```python
from build123d import *

# Parameters (mm, degrees)
BOSS_EXTRUDE1_DEPTH = 180
SKETCH3_R           = 3
SKETCH3_R_2         = 3.5
CUT_EXTRUDE1_DEPTH  = 95
SKETCH4_R           = 6
CUT_EXTRUDE2_DEPTH  = 95


with BuildPart() as part:
    # Sketch1 → Boss-Extrude1 (new body)
    with BuildSketch(Plane(origin=(0, 0, 0), x_dir=(1, 0, 0), z_dir=(0, 1, 0))):
        with BuildLine():
            Line((-20.4, 25.4), (20.4, 25.4))
            ThreePointArc((20.4, 25.4), (23.935533906, 23.935533906), (25.4, 20.4))
            Line((25.4, 20.4), (25.4, -20.4))
            ThreePointArc((25.4, -20.4), (23.935533906, -23.935533906), (20.4, -25.4))
            Line((20.4, -25.4), (-20.4, -25.4))
            ThreePointArc((-20.4, -25.4), (-23.935533906, -23.935533906), (-25.4, -20.4))
            Line((-25.4, -20.4), (-25.4, 20.4))
            ThreePointArc((-25.4, 20.4), (-23.935533906, 23.935533906), (-20.4, 25.4))
        make_face()
        with BuildLine():
            Line((-22.5, 20.4), (-22.5, -20.4))
            ThreePointArc((-22.5, -20.4), (-21.88492424, -21.88492424), (-20.4, -22.5))
            Line((-20.4, -22.5), (20.4, -22.5))
            ThreePointArc((20.4, -22.5), (21.88492424, -21.88492424), (22.5, -20.4))
            Line((22.5, -20.4), (22.5, 20.4))
            ThreePointArc((22.5, 20.4), (21.88492424, 21.88492424), (20.4, 22.5))
            Line((20.4, 22.5), (-20.4, 22.5))
            ThreePointArc((-20.4, 22.5), (-21.88492424, 21.88492424), (-22.5, 20.4))
        make_face(mode=Mode.SUBTRACT)
    extrude(amount=BOSS_EXTRUDE1_DEPTH)

    # Sketch3 → Cut-Extrude1 (cut)
    with BuildSketch(Plane.ZY.offset(25.4)):
        with Locations((-15, 67.5)):
            Circle(SKETCH3_R)
        with Locations((15, 67.5)):
            Circle(SKETCH3_R)
        with Locations((-15, 12.5)):
            Circle(SKETCH3_R_2)
        with Locations((15, 12.5)):
            Circle(SKETCH3_R)
    extrude(amount=-CUT_EXTRUDE1_DEPTH, mode=Mode.SUBTRACT)

    # Sketch4 → Cut-Extrude2 (cut)
    with BuildSketch(Plane.XY.offset(25.4)):
        with Locations((0, 31.67)):
            Circle(SKETCH4_R)
    extrude(amount=-CUT_EXTRUDE2_DEPTH, mode=Mode.SUBTRACT)


solid = part.part
```
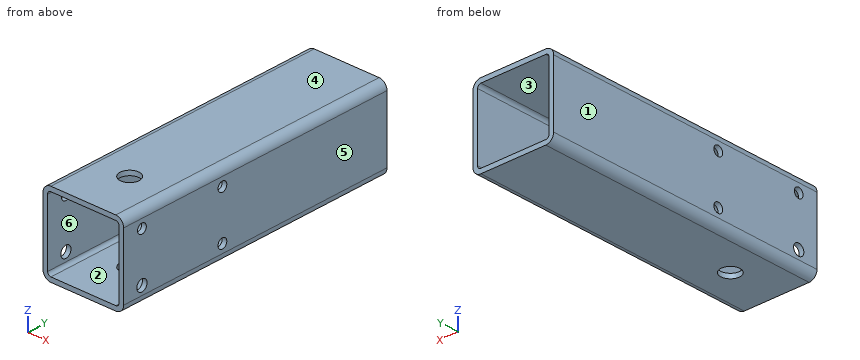
The listing builds one solid part. Answer for the finished solid, in the listing's coordinates (mm). Face numbers are marked on the shaded views. A direction names the side the tool comes from. Give positions to 0.01 mm unless a question says otherwise; leave off trailing zeros. Order: outer loops, then holes, each group sorted by start corner. A loop starts at its lowest first (then second) coordinate and runs counter-clockwise, first axis right, second up. Notation, with made-up numbers: (-7.5, 42) - (6.5, 42) arc R26 ccw to (6.5, 72) - close; hole circle Ø1 at (36.25, -4.5). An arc over 180 degrees is marked (long way). Use one line per item in the form item = value. Start each with the question number.
(1) Consider line 1 (Y direction, x = 24.65, z = -15); line 2 (Y direction, x = -24.5, z = 15); line 3 (X direction, y = 153, z = 15). Determine where each line is inside the solid, lowest interval first. Write a range as from..to.
(2) A flat-ended cylindrical pin translates along its axis: pin 1 Ø8 at (y, z) = (67.5, -15) entering from -X. Find the tip coordinate at first contact, or state that the pin passes through.
(3) For the marked faces 5 and 6, determine the directions among +Z, -Z, +X, -X, +Y, -Y from which every point of the face is accessible in a straight line to the end or side of a thin tool.
(4) A cutting plane is placed at C-C, the plane y = 12.5. State how many separate pieces and enclosed holes the cut face has, then the cut area to 3 significant figures.
(5) A cutting plane is placed at A-A, the plane z = 7. Write down the section's boundary in (x, y), then the cut area to 3 significant figures.
(6) A cutting plane is placed at B-B, the plane z = -15. Write down the section's boundary in (x, y), then the cut area to 3 significant figures.
(7) The mould has two halves that part along Z. Classify the marked faces 1, 2, 3 and 4: released by +Z, released by -Z, zero draft, split by the parting line, or undercut.
(8) A cutting plane is placed at D-D, the plane x = 0. Write down the section's boundary in (y, z).
Ans:
q1.line_1 = 0..9, 16..64.5, 70.5..180
q1.line_2 = 0..9.5, 15.5..64.5, 70.5..180
q1.line_3 = -25.4..-22.5, 22.5..25.4
q2.pin_1 = -25.4
q3.face_5 = +Z, -Z, +X, +Y, -Y
q3.face_6 = +Y, -Y
q4.separate_pieces = 4
q4.enclosed_holes = 0
q4.area = 463 mm^2
q5.outline = (-25.4, 0) - (-22.5, 0) - (-22.5, 180) - (-25.4, 180) - close; (22.5, 0) - (25.4, 0) - (25.4, 180) - (22.5, 180) - close
q5.area = 1,040 mm^2
q6.outline = (-25.4, 0) - (-22.5, 0) - (-22.5, 9) - (-25.4, 9) - close; (-25.4, 16) - (-22.5, 16) - (-22.5, 64.5) - (-25.4, 64.5) - close; (-25.4, 70.5) - (-22.5, 70.5) - (-22.5, 180) - (-25.4, 180) - close; (22.5, 0) - (25.4, 0) - (25.4, 9) - (22.5, 9) - close; (22.5, 16) - (25.4, 16) - (25.4, 64.5) - (22.5, 64.5) - close; (22.5, 70.5) - (25.4, 70.5) - (25.4, 180) - (22.5, 180) - close
q6.area = 969 mm^2
q7.face_1 = zero draft
q7.face_2 = undercut
q7.face_3 = undercut
q7.face_4 = released by +Z
q8.outline = (0, -25.4) - (25.67, -25.4) - (25.67, -22.5) - (0, -22.5) - close; (0, 22.5) - (25.67, 22.5) - (25.67, 25.4) - (0, 25.4) - close; (37.67, -25.4) - (180, -25.4) - (180, -22.5) - (37.67, -22.5) - close; (37.67, 22.5) - (180, 22.5) - (180, 25.4) - (37.67, 25.4) - close
